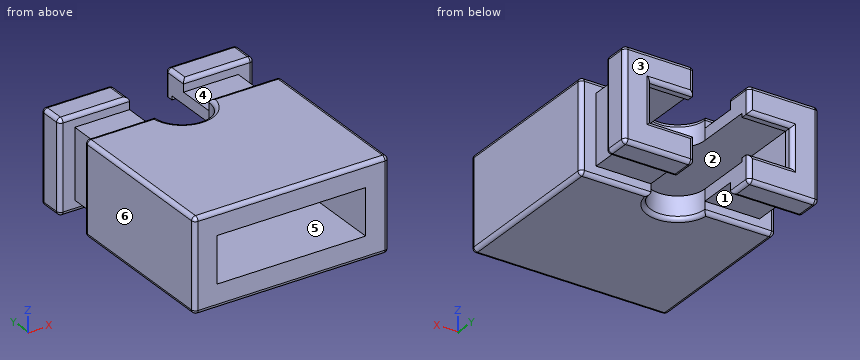
from build123d import *

# Parameters (mm, degrees)
SKETCH1_W          = 5.05
SKETCH1_H          = 5.96
MAIN_BODY_DEPTH    = 1.2
SKETCH2_W          = 5.05
SKETCH2_H          = 2.4
SKETCH2_W_2        = 4.24
SKETCH2_H_2        = 1.8
CUT_EXTRUDE1_DEPTH = 1
CUT_EXTRUDE2_START = -2.4
CUT_EXTRUDE2_DEPTH = 2.4
SKETCH4_W          = 3.85
SKETCH4_H          = 1.2
CUT_EXTRUDE3_DEPTH = 5.71
CUT_EXTRUDE4_START = -0.25
SKETCH5_W          = 3.65
SKETCH5_H          = 1
CUT_EXTRUDE4_DEPTH = 0.25
FILLET1_R          = 0.1
FILLET2_R          = 0.1


# Read off the part's stored shape, not the designer's step: Cut-Extrude2
with BuildPart() as part:
    # Sketch1 → Main Body (new, symmetric)
    with BuildSketch(Plane.XY):
        Rectangle(SKETCH1_W, SKETCH1_H)
    extrude(amount=MAIN_BODY_DEPTH, both=True)

    # Sketch2 → Cut-Extrude1 (cut)
    with BuildSketch(Plane(origin=(0, 2.28, 0), x_dir=(1, 0, 0), z_dir=(0, 1, 0))):
        Rectangle(SKETCH2_W, SKETCH2_H)
        Rectangle(SKETCH2_W_2, SKETCH2_H_2, mode=Mode.SUBTRACT)
    extrude(amount=-CUT_EXTRUDE1_DEPTH, mode=Mode.SUBTRACT)

    # Cut-Extrude2 outline → Cut-Extrude2 (cut)
    with BuildSketch(Plane.XY.offset(1.2).offset(CUT_EXTRUDE2_START)):
        with BuildLine():
            ThreePointArc((-0.7, 1.28), (0, 0.58), (0.7, 1.28))
            Line((0.7, 1.28), (0.7, 2.98))
            Line((0.7, 2.98), (-0.7, 2.98))
            Line((-0.7, 2.98), (-0.7, 1.28))
        make_face()
    extrude(amount=CUT_EXTRUDE2_DEPTH, mode=Mode.SUBTRACT)

    # Sketch4 → Cut-Extrude3 (cut)
    with BuildSketch(Plane.XZ.offset(2.98)):
        Rectangle(SKETCH4_W, SKETCH4_H)
    extrude(amount=-CUT_EXTRUDE3_DEPTH, mode=Mode.SUBTRACT)

    # Sketch5 → Cut-Extrude4 (cut)
    with BuildSketch(Plane(origin=(0, 2.98, 0), x_dir=(1, 0, 0), z_dir=(0, 1, 0)).offset(CUT_EXTRUDE4_START)):
        Rectangle(SKETCH5_W, SKETCH5_H)
    extrude(amount=CUT_EXTRUDE4_DEPTH, mode=Mode.SUBTRACT)

    # Fillet1
    fillet1_edges = [part.edges().sort_by_distance(p)[0] for p in [
        (-1.2625, 2.98, 0.5),
        (-0.7, 2.98, 0.85),
        (-1.6125, 2.98, 1.2),
        (-2.525, 2.98, 0),
        (-1.6125, 2.98, -1.2),
        (-0.7, 2.98, -0.85),
        (-1.2625, 2.98, -0.5),
        (-1.825, 2.98, 0),
        (1.2625, 2.98, -0.5),
        (0.7, 2.98, -0.85),
        (1.6125, 2.98, -1.2),
        (2.525, 2.98, 0),
        (1.6125, 2.98, 1.2),
        (0.7, 2.98, 0.85),
        (1.2625, 2.98, 0.5),
        (1.825, 2.98, 0),
        (2.525, -2.98, 0),
        (2.525, 1.28, 0),
        (-1.6125, 1.28, -1.2),
        (0, -2.98, -1.2),
        (2.525, -0.85, -1.2),
        (1.6125, 1.28, -1.2),
        (0, 0.58, -1.2),
        (1.6125, 1.28, 1.2),
        (2.525, -0.85, 1.2),
        (0, -2.98, 1.2),
        (-1.6125, 1.28, 1.2),
        (0, 0.58, 1.2),
        (-2.525, -0.85, 1.2),
        (-2.525, -2.98, 0),
        (-2.525, -0.85, -1.2),
        (-2.525, 1.28, 0),
    ]]
    fillet(fillet1_edges, radius=FILLET1_R)

    # Fillet2
    # the kernel refuses this fillet: 0.1 mm, written as the material it takes off along each edge
    with BuildSketch(Plane(origin=(-0.8, 2.88, -1.1), x_dir=(0, 0, -1), z_dir=(1, 0, 0))) as fillet2_piece_1_section:
        Polygon((0, 0), (FILLET2_R, 0), (FILLET2_R, FILLET2_R), (0, FILLET2_R), align=None)
    fillet2_piece_1 = extrude(amount=FILLET2_R, mode=Mode.PRIVATE)
    fillet2_piece_1 = fillet2_piece_1 - Plane(origin=(-0.8, 2.88, -1.1), x_dir=(0, -0.7071067811865475, 0.7071067811865475), z_dir=(1, 0, 0)) * Sphere(FILLET2_R, mode=Mode.PRIVATE)
    add(fillet2_piece_1, mode=Mode.SUBTRACT)
    with BuildSketch(Plane(origin=(-2.425, 2.88, -1.1), x_dir=(0, 0, -1), z_dir=(-1, 0, 0))) as fillet2_piece_2_section:
        Polygon((0, 0), (FILLET2_R, 0), (FILLET2_R, -FILLET2_R), (0, -FILLET2_R), align=None)
    fillet2_piece_2 = extrude(amount=FILLET2_R, mode=Mode.PRIVATE)
    fillet2_piece_2 = fillet2_piece_2 - Plane(origin=(-2.425, 2.88, -1.1), x_dir=(0, -0.7071067811865475, 0.7071067811865475), z_dir=(-1, 0, 0)) * Sphere(FILLET2_R, mode=Mode.PRIVATE)
    add(fillet2_piece_2, mode=Mode.SUBTRACT)
    with BuildSketch(Plane(origin=(-2.425, 2.88, 1.1), x_dir=(-1, 0, 0), z_dir=(0, 0, 1))) as fillet2_piece_3_section:
        Polygon((0, 0), (FILLET2_R, 0), (FILLET2_R, -FILLET2_R), (0, -FILLET2_R), align=None)
    fillet2_piece_3 = extrude(amount=FILLET2_R, mode=Mode.PRIVATE)
    fillet2_piece_3 = fillet2_piece_3 - Plane(origin=(-2.425, 2.88, 1.1), x_dir=(0.7071067811865476, -0.7071067811865475, 0), z_dir=(0, 0, 1)) * Sphere(FILLET2_R, mode=Mode.PRIVATE)
    add(fillet2_piece_3, mode=Mode.SUBTRACT)
    with BuildSketch(Plane(origin=(-0.8, 2.88, 1.1), x_dir=(0, 0, 1), z_dir=(1, 0, 0))) as fillet2_piece_4_section:
        Polygon((0, 0), (FILLET2_R, 0), (FILLET2_R, -FILLET2_R), (0, -FILLET2_R), align=None)
    fillet2_piece_4 = extrude(amount=FILLET2_R, mode=Mode.PRIVATE)
    fillet2_piece_4 = fillet2_piece_4 - Plane(origin=(-0.8, 2.88, 1.1), x_dir=(0, -0.7071067811865475, -0.7071067811865475), z_dir=(1, 0, 0)) * Sphere(FILLET2_R, mode=Mode.PRIVATE)
    add(fillet2_piece_4, mode=Mode.SUBTRACT)
    with BuildSketch(Plane(origin=(0.8, 2.88, 1.1), x_dir=(0, 0, 1), z_dir=(-1, 0, 0))) as fillet2_piece_5_section:
        Polygon((0, 0), (FILLET2_R, 0), (FILLET2_R, FILLET2_R), (0, FILLET2_R), align=None)
    fillet2_piece_5 = extrude(amount=FILLET2_R, mode=Mode.PRIVATE)
    fillet2_piece_5 = fillet2_piece_5 - Plane(origin=(0.8, 2.88, 1.1), x_dir=(0, -0.7071067811865475, -0.7071067811865475), z_dir=(-1, 0, 0)) * Sphere(FILLET2_R, mode=Mode.PRIVATE)
    add(fillet2_piece_5, mode=Mode.SUBTRACT)
    with BuildSketch(Plane(origin=(2.425, 2.88, 1.1), x_dir=(1, 0, 0), z_dir=(0, 0, 1))) as fillet2_piece_6_section:
        Polygon((0, 0), (FILLET2_R, 0), (FILLET2_R, FILLET2_R), (0, FILLET2_R), align=None)
    fillet2_piece_6 = extrude(amount=FILLET2_R, mode=Mode.PRIVATE)
    fillet2_piece_6 = fillet2_piece_6 - Plane(origin=(2.425, 2.88, 1.1), x_dir=(-0.7071067811865475, -0.7071067811865477, 0), z_dir=(0, 0, 1)) * Sphere(FILLET2_R, mode=Mode.PRIVATE)
    add(fillet2_piece_6, mode=Mode.SUBTRACT)
    with BuildSketch(Plane(origin=(2.425, 2.88, -1.1), x_dir=(1, 0, 0), z_dir=(0, 0, -1))) as fillet2_piece_7_section:
        Polygon((0, 0), (FILLET2_R, 0), (FILLET2_R, -FILLET2_R), (0, -FILLET2_R), align=None)
    fillet2_piece_7 = extrude(amount=FILLET2_R, mode=Mode.PRIVATE)
    fillet2_piece_7 = fillet2_piece_7 - Plane(origin=(2.425, 2.88, -1.1), x_dir=(-0.7071067811865475, -0.7071067811865477, 0), z_dir=(0, 0, -1)) * Sphere(FILLET2_R, mode=Mode.PRIVATE)
    add(fillet2_piece_7, mode=Mode.SUBTRACT)
    with BuildSketch(Plane(origin=(0.8, 2.88, -1.1), x_dir=(0, 0, -1), z_dir=(-1, 0, 0))) as fillet2_piece_8_section:
        Polygon((0, 0), (FILLET2_R, 0), (FILLET2_R, -FILLET2_R), (0, -FILLET2_R), align=None)
    fillet2_piece_8 = extrude(amount=FILLET2_R, mode=Mode.PRIVATE)
    fillet2_piece_8 = fillet2_piece_8 - Plane(origin=(0.8, 2.88, -1.1), x_dir=(0, -0.7071067811865475, 0.7071067811865475), z_dir=(-1, 0, 0)) * Sphere(FILLET2_R, mode=Mode.PRIVATE)
    add(fillet2_piece_8, mode=Mode.SUBTRACT)
    with BuildSketch(Plane(origin=(-2.425, 2.38, 1.1), x_dir=(0, 0, 1), z_dir=(0, -1, 0))) as fillet2_piece_9_section:
        Polygon((0, 0), (FILLET2_R, 0), (FILLET2_R, FILLET2_R), (0, FILLET2_R), align=None)
    fillet2_piece_9 = extrude(amount=FILLET2_R, mode=Mode.PRIVATE)
    fillet2_piece_9 = fillet2_piece_9 - Plane(origin=(-2.425, 2.38, 1.1), x_dir=(0.7071067811865475, 0, -0.7071067811865475), z_dir=(0, -1, 0)) * Sphere(FILLET2_R, mode=Mode.PRIVATE)
    add(fillet2_piece_9, mode=Mode.SUBTRACT)
    with BuildSketch(Plane(origin=(-2.425, 2.38, -1.1), x_dir=(0, -1, 0), z_dir=(0, 0, -1))) as fillet2_piece_10_section:
        Polygon((0, 0), (FILLET2_R, 0), (FILLET2_R, FILLET2_R), (0, FILLET2_R), align=None)
    fillet2_piece_10 = extrude(amount=FILLET2_R, mode=Mode.PRIVATE)
    fillet2_piece_10 = fillet2_piece_10 - Plane(origin=(-2.425, 2.38, -1.1), x_dir=(0.7071067811865475, 0.7071067811865477, 0), z_dir=(0, 0, -1)) * Sphere(FILLET2_R, mode=Mode.PRIVATE)
    add(fillet2_piece_10, mode=Mode.SUBTRACT)
    with BuildSketch(Plane(origin=(2.425, 2.38, -1.1), x_dir=(0, -1, 0), z_dir=(0, 0, -1))) as fillet2_piece_11_section:
        Polygon((0, 0), (FILLET2_R, 0), (FILLET2_R, -FILLET2_R), (0, -FILLET2_R), align=None)
    fillet2_piece_11 = extrude(amount=FILLET2_R, mode=Mode.PRIVATE)
    fillet2_piece_11 = fillet2_piece_11 - Plane(origin=(2.425, 2.38, -1.1), x_dir=(-0.7071067811865476, 0.7071067811865475, 0), z_dir=(0, 0, -1)) * Sphere(FILLET2_R, mode=Mode.PRIVATE)
    add(fillet2_piece_11, mode=Mode.SUBTRACT)
    with BuildSketch(Plane(origin=(2.425, 2.38, 1.1), x_dir=(0, -1, 0), z_dir=(0, 0, 1))) as fillet2_piece_12_section:
        Polygon((0, 0), (FILLET2_R, 0), (FILLET2_R, FILLET2_R), (0, FILLET2_R), align=None)
    fillet2_piece_12 = extrude(amount=FILLET2_R, mode=Mode.PRIVATE)
    fillet2_piece_12 = fillet2_piece_12 - Plane(origin=(2.425, 2.38, 1.1), x_dir=(-0.7071067811865476, 0.7071067811865475, 0), z_dir=(0, 0, 1)) * Sphere(FILLET2_R, mode=Mode.PRIVATE)
    add(fillet2_piece_12, mode=Mode.SUBTRACT)
    with BuildSketch(Plane(origin=(-0.7, 2.88, 1.2), x_dir=(0, 0, -1), z_dir=(0, -1, 0)), Plane(origin=(0.7, 2.03, 1.2), x_dir=(0, 0, -1), z_dir=(0, 1, 0))) as fillet2_piece_13:
        with BuildLine():
            CenterArc((FILLET2_R, -FILLET2_R), FILLET2_R, 90, 90)
            Line((0, -FILLET2_R), (0, 0))
            Line((0, 0), (FILLET2_R, 0))
        make_face()
    extrude(amount=0.85, mode=Mode.SUBTRACT)
    with BuildSketch(Plane(origin=(-2.525, 2.38, 1.2), x_dir=(1, 0, 0), z_dir=(0, 1, 0)), Plane(origin=(-2.525, 2.38, -1.2), x_dir=(0, 0, 1), z_dir=(0, 1, 0)), Plane(origin=(2.525, 2.88, 1.2), x_dir=(-1, 0, 0), z_dir=(0, -1, 0))) as fillet2_piece_14:
        with BuildLine():
            CenterArc((FILLET2_R, FILLET2_R), FILLET2_R, 180, 90)
            Line((0, FILLET2_R), (0, 0))
            Line((0, 0), (FILLET2_R, 0))
        make_face()
    extrude(amount=0.5, mode=Mode.SUBTRACT)
    with BuildSketch(Plane(origin=(2.525, 2.88, -1.2), x_dir=(-1, 0, 0), z_dir=(0, -1, 0))) as fillet2_piece_15:
        with BuildLine():
            CenterArc((FILLET2_R, -FILLET2_R), FILLET2_R, 90, 90)
            Line((0, -FILLET2_R), (0, 0))
            Line((0, 0), (FILLET2_R, 0))
        make_face()
    extrude(amount=0.5, mode=Mode.SUBTRACT)
    with BuildSketch(Plane(origin=(0.7, 2.03, -1.2), x_dir=(0, 0, 1), z_dir=(0, 1, 0)), Plane(origin=(-0.7, 2.88, -1.2), x_dir=(0, 0, 1), z_dir=(0, -1, 0))) as fillet2_piece_16:
        with BuildLine():
            CenterArc((FILLET2_R, FILLET2_R), FILLET2_R, 180, 90)
            Line((0, FILLET2_R), (0, 0))
            Line((0, 0), (FILLET2_R, 0))
        make_face()
    extrude(amount=0.85, mode=Mode.SUBTRACT)
    with BuildSketch(Plane(origin=(2.525, 2.28, 1.1), x_dir=(-1, 0, 0), z_dir=(0, 0, -1))) as fillet2_piece_17:
        with BuildLine():
            CenterArc((FILLET2_R, FILLET2_R), FILLET2_R, 180, 90)
            Line((0, FILLET2_R), (0, 0))
            Line((0, 0), (FILLET2_R, 0))
        make_face()
    extrude(amount=2.2, mode=Mode.SUBTRACT)
    with BuildSketch(Plane(origin=(2.425, 2.28, -1.2), x_dir=(0, 0, 1), z_dir=(-1, 0, 0))) as fillet2_piece_18:
        with BuildLine():
            CenterArc((FILLET2_R, FILLET2_R), FILLET2_R, 180, 90)
            Line((0, FILLET2_R), (0, 0))
            Line((0, 0), (FILLET2_R, 0))
        make_face()
    extrude(amount=1.975, mode=Mode.SUBTRACT)
    with BuildSketch(Plane(origin=(-2.525, 2.28, -1.1), x_dir=(0, 1, 0), z_dir=(0, 0, 1))) as fillet2_piece_19:
        with BuildLine():
            CenterArc((FILLET2_R, -FILLET2_R), FILLET2_R, 90, 90)
            Line((0, -FILLET2_R), (0, 0))
            Line((0, 0), (FILLET2_R, 0))
        make_face()
    extrude(amount=2.2, mode=Mode.SUBTRACT)
    with BuildSketch(Plane(origin=(-2.425, 2.28, 1.2), x_dir=(0, 1, 0), z_dir=(1, 0, 0)), Plane(origin=(-0.45, 2.28, -1.2), x_dir=(0, 1, 0), z_dir=(-1, 0, 0)), Plane(origin=(0.45, 2.28, 1.2), x_dir=(0, 1, 0), z_dir=(1, 0, 0))) as fillet2_piece_20:
        with BuildLine():
            CenterArc((FILLET2_R, -FILLET2_R), FILLET2_R, 90, 90)
            Line((0, -FILLET2_R), (0, 0))
            Line((0, 0), (FILLET2_R, 0))
        make_face()
    extrude(amount=1.975, mode=Mode.SUBTRACT)


solid = part.part
Could you check a few things on this model? Use its own coordinates, in mm. Face numbers are marked on the shaded views. A direction names the side the tool comes from. Coordinates: 2 decimals unless noted, no trailing zeros. Write each loop counter-clockwise with the first axis right and the second up, starting at its lowest first coordinate (ties: lowest second). Pieces come first, ordered by that corner, then holes. Notation, with made-up numbers: M -26,57.25 L -16,57.25 A26 ccw -16,74.25 Z; hole C 52.25,51 d3. An arc over 180 degrees is marked long. One line per question, with ' | ' between items.
1) For the marked faces 1, 2 and 3, which set-ups out of +Z, -Z, +X, -X, +Y, -Y let a thin tool reach every point of the face, with its end or its side?
Checks:
face 1: -Z, +X, -X | face 2: -Y | face 3: +Z, -Z, +X, -X, +Y
2) For pin 1 Ø0.5 at (y, z) = (2, 1) entering from -X; pin 2 Ø0.5 at (x, y) = (1.5, 2) entering from +Z; pin 3 Ø0.5 at (y, z) = (2, -0.5) entering from +X; pin 4 Ø1.4 at (x, z) = (1.5, -0.5) entering from -Y, each with a flat end and sliding along its axis, tell me the tip position at first contact or that it passes through.
Checks:
pin 1: x = -2.12 | pin 2: z = 0.9 | pin 3: x = 2.12 | pin 4: y = -2.98
3) I need wall thicknesses on probe 1 along X at (y, z) = (2.5, -0.55) (3 decimals); probe 2 along X at (y, z) = (1.9, -0.05) (3 decimals); probe 3 along Y at (x, z) = (2.15, -0.6). Which ranges of each line are inside material? Lowest first, please. Write a range as [from, to].
Checks:
probe 1: [-2.525, -1.925], [1.925, 2.525] | probe 2: [-2.12, -1.925], [1.925, 2.12] | probe 3: [-2.98, 1.28], [2.28, 2.98]
4) If we mould it in two halves opening along Z, with no side actions, what happens to the marked faces 4, 5 and 6? For each: released by +Z, released by -Z, zero draft, split by the parting line, or undercut.
Checks:
face 4: released by +Z | face 5: undercut | face 6: zero draft
5) Imagine slicing it at B-B, the plane y = -0.4. Write out the boundary of the cut face in (x, z) (3 decimals).
Checks:
outline: M -2.525,-1.1 A0.1 ccw -2.425,-1.2 L 2.425,-1.2 A0.1 ccw 2.525,-1.1 L 2.525,1.1 A0.1 ccw 2.425,1.2 L -2.425,1.2 A0.1 ccw -2.525,1.1 Z; hole M -1.925,-0.6 L 1.925,-0.6 L 1.925,0.6 L -1.925,0.6 Z
6) Imagine slicing it at A-A, the plane x = 0. Write out the boundary of the cut face in (y, z).
Checks:
outline: M -2.98,-1.1 A0.1 ccw -2.88,-1.2 L 0.48,-1.2 A0.1 ccw 0.58,-1.1 L 0.58,-0.6 L -2.98,-0.6 Z; M -2.98,0.6 L 0.58,0.6 L 0.58,1.1 A0.1 ccw 0.48,1.2 L -2.88,1.2 A0.1 ccw -2.98,1.1 Z
